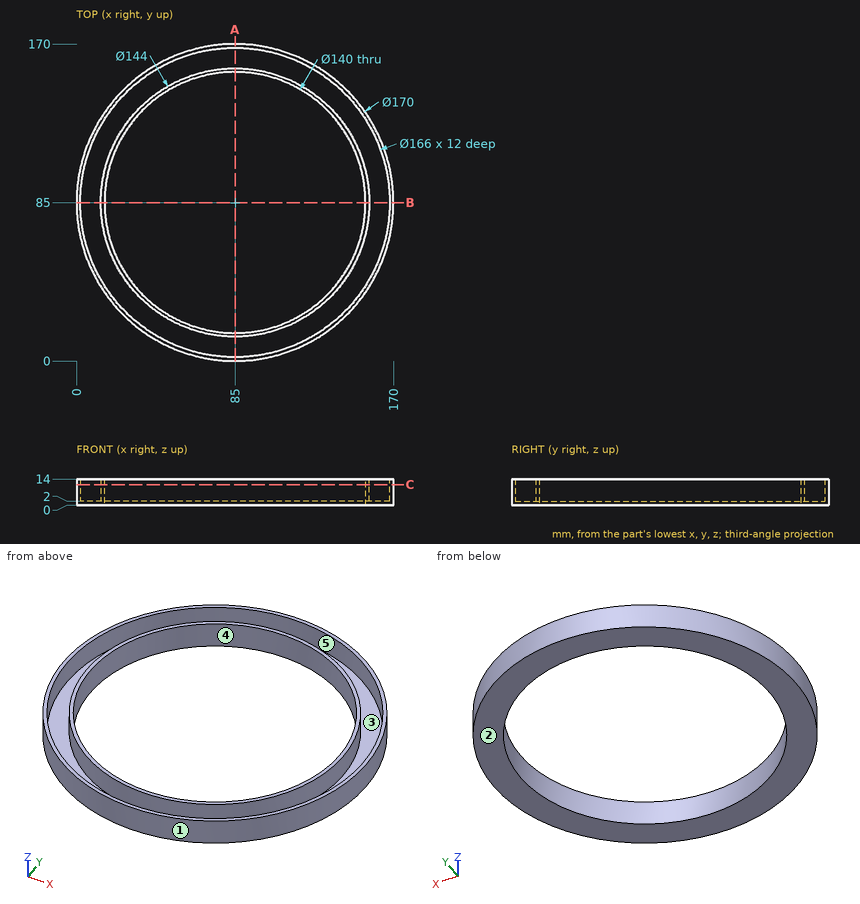
Can you work these out from the drawing? Everything is in mm from the part's minimum corner. A direction names the side the tool comes from. Coordinates: 2 decimals unless noted, no trailing zeros. Loops run counter-clockwise (first coordinate to the right, second up) from the corner with the lowest first, then second, coordinate; pieces in that order, holes last. Notation, with made-up numbers: (71, 51.5) - (115, 51.5) arc R37 ccw to (115, 87.5) - close; hole circle Ø1 at (81.25, 68.25). An arc over 180 degrees is marked (long way). Use a Markdown table: item, result.
Item 1: For the marked faces 4 and 5, which set-ups out of +Z, -Z, +X, -X, +Y, -Y let a thin tool reach every point of the face, with its end or its side?
Numbers:
| item | result |
|---|---|
| face 4 | +Z, -Z |
| face 5 | +Z |
Item 2: I want a section at A-A on x = 85. Please give me the cut outline in (y, z), and give its area (3 significant figures).
Numbers:
| item | result |
|---|---|
| outline | (0, 0) - (15, 0) - (15, 14) - (13, 14) - (13, 2) - (2, 2) - (2, 14) - (0, 14) - close; (155, 0) - (170, 0) - (170, 14) - (168, 14) - (168, 2) - (157, 2) - (157, 14) - (155, 14) - close |
| area | 156 mm2 |
Item 3: I want a section at C-C on z = 11. Please give me the cut outline in (x, y).
Numbers:
| item | result |
|---|---|
| outline | circle Ø170 at (85, 85); circle Ø144 at (85, 85); hole circle Ø166 at (85, 85); hole circle Ø140 at (85, 85) |
Item 4: Will these pins go through, and if not, where does the flat tip stop? pin 1 (3 mm diameter, centred on x = 145.5, z = 8, fed in from -Y); pin 2 (6 mm diameter, centred on x = 21, z = 5, fed in from +Y); pin 3 (8 mm diameter, centred on y = 28, z = 1.5, fed in from -X).
Numbers:
| item | result |
|---|---|
| pin 1 | stops at y = 23.81 |
| pin 2 | stops at y = 144.19 |
| pin 3 | stops at x = 18.55 |
Item 5: We'd pull the mould along X, two halves only. Please class the marked faces 1, 2 and 3: released by +X, released by -X, zero draft, split by the parting line, or undercut.
Numbers:
| item | result |
|---|---|
| face 1 | split by the parting line |
| face 2 | zero draft |
| face 3 | undercut |
Item 6: If I drill on probe 1 along Y at (x, z) = (85, 5.75); probe 2 along Y at (x, z) = (103, 13); probe 3 along X at (y, z) = (53, 5), over which ranges is the centre line in solid material (lowest first)? Write a range as from..to.
Numbers:
| item | result |
|---|---|
| probe 1 | y = 0..2, 13..15, 155..157, 168..170 |
| probe 2 | y = 1.93..3.98, 15.29..17.35, 152.65..154.71, 166.02..168.07 |
| probe 3 | x = 6.25..8.42, 20.5..22.74, 147.26..149.5, 161.58..163.75 |
